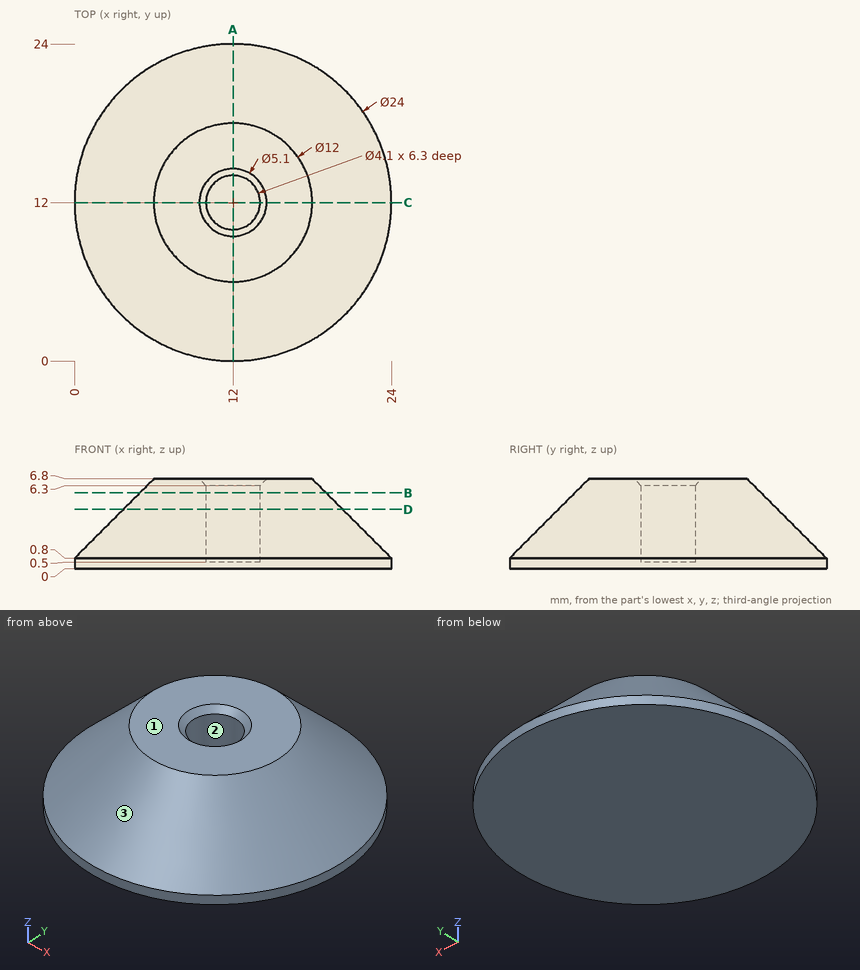
Verification items for this drawing (mm, ordinates from the low corner). Coordinates: 2 decimals unless noted, no trailing zeros. Write each loop counter-clockwise with the first axis right and the second up, starting at its lowest first coordinate (ties: lowest second). Pieces come first, ordered by that corner, then holes. Notation, with made-up numbers: M 2,78.25 L 44,78.25 A27 cw 44,96.25 Z; hole C -22,38.5 d7. An arc over 180 degrees is marked long. Answer as a JSON object with one key per item and string values. Group by question number.
(1) Gauge pin test, flat ends, axial feed: pin 1 (3 mm diameter, centred on y = 5.5, z = 2.5, fed in from -X); pin 2 (1.5 mm diameter, centred on x = 10, z = 1.5, fed in from +Y); pin 3 (3.5 mm diameter, centred on x = 11.5, y = 11.5, fed in from +Z). Record the tip position at first contact, or that the pin passes through.
(2) Cross-section at B-B, the plane z = 5.75. Record the cut outline in (x, y).
(3) Material ranges on line 1 (Y direction, x = 12, z = 3.45); line 2 (Z direction, x = 12.25, y = 12.25); line 3 (Y direction, x = 13.5, z = 2), recorded low to high.
(4) Cross-section at A-A, the plane x = 12. Record the cut outline in (y, z).
(5) Release check for a two-part mould opening along X. For the marked faces 1, 2 and 3 record: +X half, -X half, draft (parallel to the pull), parting line (faces both ways), or undercut.
(6) Cross-section at D-D, the plane z = 4.5. Record the cut outline in (x, y), and give its area (3 significant figures).
Reply:
{
 "1": {"pin 1": "x = 1.92", "pin 2": "y = 23.87", "pin 3": "z = 6.71"},
 "2": {"outline": "C 12,12 d14.1; hole C 12,12 d4.1"},
 "3": {"line 1": "2.65 to 9.95, 14.05 to 21.35", "line 2": "0 to 0.5", "line 3": "1.3 to 10.6, 13.4 to 22.7"},
 "4": {"outline": "M 0,0 L 24,0 L 24,0.8 L 18,6.8 L 14.55,6.8 L 14.05,6.3 L 14.05,0.5 L 9.95,0.5 L 9.95,6.3 L 9.45,6.8 L 6,6.8 L 0,0.8 Z"},
 "5": {"face 1": "draft", "face 2": "undercut", "face 3": "parting line"},
 "6": {"outline": "C 12,12 d16.6; hole C 12,12 d4.1", "area": "203 mm²"}
}
